The model under review builds one solid part; all positions refer to its coordinate system, in mm. A direction names the side the tool comes from. Give positions to 0.01 mm unless a question says otherwise; leave off trailing zeros. Loops run counter-clockwise (first coordinate to the right, second up) from the corner with the lowest first, then second, coordinate; pieces in that order, holes last. Notation, with made-up numbers: (81.25, 60) - (129.25, 60) arc R30 cw to (129.25, 98) - close; hole circle Ø3 at (69.25, 12.25). An arc over 180 degrees is marked (long way). Answer as a JSON object with one key per item and string values.
from build123d import *

# Parameters (mm, degrees)
BOSS_EXTRUDE1_DEPTH   = 140
SKETCH4_W             = 25
SKETCH4_H             = 27
BOSS_EXTRUDE2_DEPTH   = 5
SKETCH5_W             = 25
SKETCH5_H             = 27
BOSS_EXTRUDE3_DEPTH   = 5
FILLET1_R             = 2
SKETCH6_R             = 1.75
SKETCH6_R_2           = 1.8
CUT_EXTRUDE1_DEPTH    = 137
CHAMFER1_SIZE         = 1.5
CHAMFER1_SIZE2        = 2.5
CHAMFER2_SIZE         = 2.5
CHAMFER2_SIZE2        = 1.5
CHAMFER2_PART_2_SIZE  = 2.5
CHAMFER2_PART_2_SIZE2 = 1.5
SKETCH8_R             = 4
CUT_EXTRUDE2_DEPTH    = 50


with BuildPart() as part:
    # Sketch3 → Boss-Extrude1 (new body)
    with BuildSketch(Plane.XY):
        Polygon((-58, 0), (58, 0), (58, -32), (68, -32), (68, -49), (63, -49), (63, -37), (53, -37), (53, -5), (-53, -5), (-53, -37), (-63, -37), (-63, -49), (-68, -49), (-68, -32), (-58, -32), align=None)
    extrude(amount=-BOSS_EXTRUDE1_DEPTH)

    # Sketch4 → Boss-Extrude2 (add)
    with BuildSketch(Plane.XY):
        with Locations((40.5, -18.5)):
            Rectangle(SKETCH4_W, SKETCH4_H)
    extrude(amount=-BOSS_EXTRUDE2_DEPTH)

    # Sketch5 → Boss-Extrude3 (add)
    with BuildSketch(Plane(origin=(0, 0, -140), x_dir=(-1, 0, 0), z_dir=(0, 0, -1))):
        with Locations((40.5, -18.5)):
            Rectangle(SKETCH5_W, SKETCH5_H)
    extrude(amount=-BOSS_EXTRUDE3_DEPTH)

    # Fillet1
    fillet1_edges = [part.edges().sort_by_distance(p)[0] for p in [
        (-58, -16, -140),
        (63, -32, 0),
        (68, -40.5, 0),
        (-63, -32, -140),
        (-68, -40.5, 0),
        (-63, -32, 0),
        (-68, -40.5, -140),
        (-58, -16, 0),
        (0, 0, 0),
        (58, -16, 0),
        (58, -32, -70),
        (68, -32, -70),
        (68, -49, -70),
        (-68, -49, -70),
        (-68, -32, -70),
        (-58, -32, -70),
        (-58, 0, -70),
        (58, 0, -70),
        (58, -16, -140),
        (68, -40.5, -140),
        (63, -32, -140),
        (0, 0, -140),
    ]]
    fillet(fillet1_edges, radius=FILLET1_R)

    # Sketch6 → Cut-Extrude1 (cut, through all)
    with BuildSketch(Plane(origin=(68, 0, 0), x_dir=(0, 0, -1), z_dir=(1, 0, 0))):
        with Locations((22, -43)):
            Circle(SKETCH6_R)
        with Locations((118, -43)):
            Circle(SKETCH6_R_2)
    extrude(amount=-CUT_EXTRUDE1_DEPTH, mode=Mode.SUBTRACT)

    # Chamfer1
    chamfer1_edges = [part.edges().sort_by_distance(p)[0] for p in [
        (68, -43, -20.25),
        (68, -43, -116.2),
    ]]
    chamfer1_side = [part.faces().sort_by_distance(p)[0] for p in [
        (68, -40.471685324, -69.984689184),
    ]]
    chamfer(chamfer1_edges, length=CHAMFER1_SIZE, length2=CHAMFER1_SIZE2, reference=chamfer1_side[0])

    # Chamfer2
    chamfer2_edges = [part.edges().sort_by_distance(p)[0] for p in [
        (-68, -43, -20.25),
    ]]
    chamfer2_side = [part.faces().sort_by_distance(p)[0] for p in [
        (-65.5, -43, -20.25),
    ]]
    chamfer(chamfer2_edges, length=CHAMFER2_SIZE, length2=CHAMFER2_SIZE2, reference=chamfer2_side[0])

    # Chamfer2 part 2
    chamfer2_part_2_edges = [part.edges().sort_by_distance(p)[0] for p in [
        (-68, -43, -116.2),
    ]]
    chamfer2_part_2_side = [part.faces().sort_by_distance(p)[0] for p in [
        (-65.5, -43, -116.2),
    ]]
    chamfer(chamfer2_part_2_edges, length=CHAMFER2_PART_2_SIZE, length2=CHAMFER2_PART_2_SIZE2, reference=chamfer2_part_2_side[0])

    # Sketch8 → Cut-Extrude2 (cut, through all)
    with BuildSketch(Plane(origin=(0, 0, 0), x_dir=(1, 0, 0), z_dir=(0, 1, 0))):
        with Locations((0, 90)):
            Circle(SKETCH8_R)
        with Locations((0, 50)):
            Circle(SKETCH8_R)
    extrude(amount=-CUT_EXTRUDE2_DEPTH, mode=Mode.SUBTRACT)


solid = part.part
Q1. Clearance check with flat-ended pins moving along their axes: pin 1 Ø2 at (y, z) = (-17.5, -121.5) entering from -X; pin 2 Ø1.8 at (x, z) = (62, -45) entering from +Y; pin 3 Ø5 at (x, z) = (-56.5, -50.5) entering from -Y; pin 4 Ø2 at (y, z) = (-43, -22) entering from +X. State where each tip first meets the part, or that it passes through.
Results:
{"pin 1": "stops at x = -58", "pin 2": "stops at y = -32", "pin 3": "stops at y = -37", "pin 4": "passes through"}
Q2. Consider section A-A, the plane z = -90. State the section outline as (x, y) points, plus the area to 3 significant figures.
Results:
{"outline": "(-68, -47) arc R2 ccw to (-66, -49) - (-63, -49) - (-63, -37) - (-53, -37) - (-53, -5) - (-4, -5) - (-4, 0) - (-56, 0) arc R2 ccw to (-58, -2) - (-58, -30) arc R2 cw to (-60, -32) - (-66, -32) arc R2 ccw to (-68, -34) - close; (4, -5) - (53, -5) - (53, -37) - (63, -37) - (63, -49) - (66, -49) arc R2 ccw to (68, -47) - (68, -34) arc R2 ccw to (66, -32) - (60, -32) arc R2 cw to (58, -30) - (58, -2) arc R2 ccw to (56, 0) - (4, 0) - close", "area": "1,080 mm^2"}
Q3. For faces 1 (the face through (63, -32, -69)), 2 (the face through (-53, -21, -69)), 3 (the face through (40, -18, -5)), 4 (the face through (-58, -16, -69)), 5 (the face through (28, -19, -2)), list the 3-axis set-ups (+Z, -Z, +X, -X, +Y, -Y) from which the entire face can be reached by the end or side of a thin tool; tool diameter is ignored.
Results:
{"face 1": "+Z, -Z, +X, +Y", "face 2": "+Z, -Y", "face 3": "-Z, -Y", "face 4": "+Z, -Z, -X, +Y", "face 5": "+Z, -Z, -Y"}
Q4. Consider section D-D, the plane x = 33. State the section outline as (y, z) points, plus the area to 3 significant figures.
Results:
{"outline": "(-32, -5) - (-5, -5) - (-5, -140) - (-2, -140) arc R2 ccw to (0, -138) - (0, -2) arc R2 ccw to (-2, 0) - (-32, 0) - close", "area": "833 mm^2"}
Q5. The part is to be moulded in two halves that separate along Z. For faces 6 (the face through (64.268, -41.783, -116.673)), 7 (the face through (29, -18, 0)), 8 (the face through (63, -43, -69)), say which applies: +Z half, -Z half, draft (parallel to the pull), parting line (faces both ways), or undercut.
Results:
{"face 6": "undercut", "face 7": "+Z half", "face 8": "draft"}
Q6. To check wall thickness, follow probe 1 along Z at (x, y) = (0, -3); probe 2 along Y at (x, z) = (-64.8, -22); probe 3 along X at (y, z) = (-19.5, -62.5). State the ranges of each line that lie inside material, in increasing order. Write a range as [from, to].
Results:
{"probe 1": "z = [-140, -94], [-86, -54], [-46, 0]", "probe 2": "y = [-49, -44.75], [-41.25, -32]", "probe 3": "x = [-58, -53], [53, 58]"}
Q7. Consider section B-B, the plane x = 0. State the section outline as (y, z) points.
Results:
{"outline": "(-5, -140) - (-2, -140) arc R2 ccw to (0, -138) - (0, -94) - (-5, -94) - close; (-5, -86) - (0, -86) - (0, -54) - (-5, -54) - close; (-5, -46) - (0, -46) - (0, -2) arc R2 ccw to (-2, 0) - (-5, 0) - close"}
Q8. Consider section C-C, the plane y = -21. State the section outline as (x, z) points.
Results:
{"outline": "(-58, -138) arc R2 ccw to (-56, -140) - (-28, -140) - (-28, -135) - (-53, -135) - (-53, 0) - (-56, 0) arc R2 ccw to (-58, -2) - close; (28, -5) - (53, -5) - (53, -140) - (56, -140) arc R2 ccw to (58, -138) - (58, -2) arc R2 ccw to (56, 0) - (28, 0) - close"}
